Part model, mm, in its own coordinate system. A direction names the side the tool comes from. Round coordinates to 2 decimals unless told otherwise and drop trailing zeros. Loops run counter-clockwise (first coordinate to the right, second up) from the corner with the lowest first, then second, coordinate; pieces in that order, holes last. Notation, with made-up numbers: M 31,84 L 57,84 A15 cw 57,100 Z; hole C 74.5,-31.75 d3. An arc over 180 degrees is marked long. Answer as CSV lines item,"result". Start each with the question number.
Item 1: Which spindle directions (+Z, -Z, +X, -X, +Y, -Y) get a long thin tool onto all of the face, cutting with end or side? Do faces 1 (the flat face through (346.075, 3, -181)), 2 (the flat face through (374.65, 3, -31)), 3 (the flat face through (365.125, 3, -181)), 4 (the flat face through (273, 3, -184.15)), 5 (the flat face through (3, 3, -92.075)). Say none if no direction does.
Item 2: Drop flat-ended pins along their axis: pin 1 Ø3 at (x, y) = (377.5, 2) entering from +Z; pin 2 Ø0.9 at (y, z) = (4, -30) entering from +X; pin 3 Ø2.5 at (x, y) = (8, 3.5) entering from -Z; pin 4 Ø3 at (y, z) = (1.5, -179.5) entering from -X (3 decimals). Give the stop position or say it passes through.
Item 3: Band-saw the part on A-A (x = 79). Give the cut face in (y, z).
Item 4: Wall check: line 1 (Z direction, x = 107.95, y = 3.25); line 2 (Z direction, x = 364.5, y = 2.75); line 3 (X direction, y = 5.25, z = -114.3). Give the ranges that are in metal, low to high.
Item 5: Mould opens along X. For faces 6 (the flat face through (149, 3, -177.8)), 7 (the flat face through (263.525, 3, -181)), 8 (the flat face through (188, 3, 0)), 9 (the flat face through (374.65, 3, -19)) say: pulls with the +X half, pulls with the -X half, needs draft (parallel to the pull), parting line crosses it, or undercut.
Item 6: Band-saw the part on B-B (y = 4.75). Count the separate pieces of the cut face and the enclosed holes in it, and give its area (3 significant figures).
```python
from build123d import *

# Parameters (mm, degrees)
SKETCH1_W                    = 381
SKETCH1_H                    = 177.8
BOSS_EXTRUDE1_DEPTH          = 6.35
SKETCH2_W                    = 19.05
SKETCH2_H                    = 6.35
BOSS_EXTRUDE2_DEPTH          = 6.35
F_10_0_1935_DIAMETER_HOLE1_D = 4.9149
LPATTERN1_COUNT              = 5
LPATTERN1_PITCH              = 82.55
CUT_EXTRUDE2_DEPTH           = 424.216900655
LPATTERN4_COUNT              = 3
LPATTERN4_PITCH              = 57.15
SKETCH8_R                    = 2.413
CUT_EXTRUDE3_DEPTH           = 424.216900655


with BuildPart() as part:
    # Sketch1 → Boss-Extrude1 (new body)
    with BuildSketch(Plane(origin=(0, 0, 0), x_dir=(1, 0, 0), z_dir=(0, 1, 0))):
        with Locations((190.5, 88.9)):
            Rectangle(SKETCH1_W, SKETCH1_H)
    extrude(amount=BOSS_EXTRUDE1_DEPTH)

    # Sketch2 → Boss-Extrude2 (add)
    with BuildSketch(Plane(origin=(0, 6.35, 0), x_dir=(1, 0, 0), z_dir=(0, 1, 0))):
        with Locations((25.4, 180.975)):
            Rectangle(SKETCH2_W, SKETCH2_H)
    boss_extrude2 = extrude(amount=-BOSS_EXTRUDE2_DEPTH)

    # #10 (0.1935) Diameter Hole1 (through all)
    with Locations(Plane(origin=(0, 6.35, 0), x_dir=(1, 0, 0), z_dir=(0, 1, 0))):
        with Locations((25.4, 180.975)):
            f_10_0_1935_diameter_hole1 = Hole(F_10_0_1935_DIAMETER_HOLE1_D / 2)

    # LPattern1: Boss-Extrude2, #10 (0.1935) Diameter Hole1 ×5
    with Locations(*[(i * LPATTERN1_PITCH, 0, 0) for i in range(1, LPATTERN1_COUNT)]):
        add(boss_extrude2)
        add(f_10_0_1935_diameter_hole1, mode=Mode.SUBTRACT)

    # Sketch7 → Cut-Extrude2 (cut, through all)
    with BuildSketch(Plane(origin=(0, 6.35, 0), x_dir=(1, 0, 0), z_dir=(0, 1, 0))):
        Polygon((0, 34.925), (0, 15.875), (6.35, 15.875), (6.35, 22.86), (11.049, 22.86), (11.049, 19.9009), (14.351, 19.9009), (14.351, 22.86), (19.05, 22.86), (19.05, 27.94), (14.351, 27.94), (14.351, 30.8991), (11.049, 30.8991), (11.049, 27.94), (6.35, 27.94), (6.35, 34.925), align=None)
    cut_extrude2 = extrude(amount=-CUT_EXTRUDE2_DEPTH, mode=Mode.SUBTRACT)

    # Mirror2: Cut-Extrude2 across plane
    add(cut_extrude2.mirror(Plane.ZY.offset(-190.5)), mode=Mode.SUBTRACT)

    # LPattern4: Cut-Extrude2 ×3
    with Locations(*[(0, 0, -i * LPATTERN4_PITCH) for i in range(1, LPATTERN4_COUNT)]):
        add(cut_extrude2, mode=Mode.SUBTRACT)

    # Sketch8 → Cut-Extrude3 (cut, through all)
    with BuildSketch(Plane(origin=(0, 6.35, 0), x_dir=(1, 0, 0), z_dir=(0, 1, 0))):
        with Locations(Location((374.65, 165.1, 0), (0, 0, 270))):
            Circle(SKETCH8_R)
        with Locations(Location((374.65, 139.7, 0), (0, 0, 270))):
            Circle(SKETCH8_R)
        with Locations(Location((374.65, 114.3, 0), (0, 0, 270))):
            Circle(SKETCH8_R)
        with Locations(Location((374.65, 88.9, 0), (0, 0, 270))):
            Circle(SKETCH8_R)
        with Locations(Location((374.65, 63.5, 0), (0, 0, 270))):
            Circle(SKETCH8_R)
    extrude(amount=-CUT_EXTRUDE3_DEPTH, mode=Mode.SUBTRACT)


solid = part.part
```
Answer block:
1,face 1,"-Z, +Y, -Y"
1,face 2,"+X, +Y, -Y"
1,face 3,"-Z, +X, +Y, -Y"
1,face 4,"-Z, +X, -X, +Y, -Y"
1,face 5,"-X, +Y, -Y"
2,pin 1,"stops at z = 0"
2,pin 2,"stops at x = 374.65"
2,pin 3,"stops at z = -177.8"
2,pin 4,"stops at x = 15.875"
3,outline,"M 0,-177.8 L 6.35,-177.8 L 6.35,0 L 0,0 Z"
4,line 1,"z = -184.15 to -183.43, -178.52 to 0"
4,line 2,"z = -184.15 to -27.94, -22.86 to 0"
4,line 3,"x = 0 to 372.24, 377.06 to 381"
5,face 6,"undercut"
5,face 7,"undercut"
5,face 8,"needs draft"
5,face 9,"pulls with the +X half"
6,separate pieces,"1"
6,enclosed holes,"10"
6,area,"67,300 mm^2"
